Source: CAD feature listing. Evaluate the final solid. Frame: model axes, mm. A direction names the side the tool comes from. Round coordinates to 2 decimals unless told otherwise and drop trailing zeros. Order: outer loops, then holes, each group sorted by start corner. A loop starts at its lowest first (then second) coordinate and runs counter-clockwise, first axis right, second up. Notation, with made-up numbers: M 78,-26.75 L 114,-26.75 A13 cw 114,-14.75 Z; hole C 66.25,74.5 d6. An arc over 180 degrees is marked long. Use CSV: the item, a comma, the result in double quotes. Start each with the question number.
```python
from build123d import *

# Parameters (mm, degrees)
SKETCH1_W           = 24
SKETCH1_H           = 24
SKETCH1_R           = 2.1
BOSS_EXTRUDE1_DEPTH = 2
SKETCH2_W           = 24
SKETCH2_H           = 26
SKETCH2_R           = 2
BOSS_EXTRUDE2_DEPTH = 2


with BuildPart() as part:
    # Sketch1 → Boss-Extrude1 (new body)
    with BuildSketch(Plane(origin=(0, 0, 0), x_dir=(1, 0, 0), z_dir=(0, 1, 0))):
        with Locations((12, 0)):
            Rectangle(SKETCH1_W, SKETCH1_H)
        with Locations(Location((4, 8, 0), (0, 0, 270))):
            Circle(SKETCH1_R, mode=Mode.SUBTRACT)
        with Locations(Location((12, 8, 0), (0, 0, 270))):
            Circle(SKETCH1_R, mode=Mode.SUBTRACT)
        with Locations(Location((20, 8, 0), (0, 0, 270))):
            Circle(SKETCH1_R, mode=Mode.SUBTRACT)
        with Locations(Location((12, 0, 0), (0, 0, 270))):
            Circle(SKETCH1_R, mode=Mode.SUBTRACT)
        with Locations(Location((20, 0, 0), (0, 0, 270))):
            Circle(SKETCH1_R, mode=Mode.SUBTRACT)
        with Locations(Location((12, -8, 0), (0, 0, 270))):
            Circle(SKETCH1_R, mode=Mode.SUBTRACT)
        with Locations(Location((20, -8, 0), (0, 0, 270))):
            Circle(SKETCH1_R, mode=Mode.SUBTRACT)
        with Locations(Location((4, 0, 0), (0, 0, 270))):
            Circle(SKETCH1_R, mode=Mode.SUBTRACT)
        with Locations(Location((4, -8, 0), (0, 0, 270))):
            Circle(SKETCH1_R, mode=Mode.SUBTRACT)
    extrude(amount=BOSS_EXTRUDE1_DEPTH)

    # Sketch2 → Boss-Extrude2 (add)
    with BuildSketch(Plane.ZY):
        with Locations((0, 13)):
            Rectangle(SKETCH2_W, SKETCH2_H)
        with Locations((-8, 21.666666667)):
            Circle(SKETCH2_R, mode=Mode.SUBTRACT)
        with Locations((0, 21.666666667)):
            Circle(SKETCH2_R, mode=Mode.SUBTRACT)
        with Locations((8, 21.666666667)):
            Circle(SKETCH2_R, mode=Mode.SUBTRACT)
        with Locations((0, 13.666666667)):
            Circle(SKETCH2_R, mode=Mode.SUBTRACT)
        with Locations((8, 13.666666667)):
            Circle(SKETCH2_R, mode=Mode.SUBTRACT)
        with Locations((0, 5.666666667)):
            Circle(SKETCH2_R, mode=Mode.SUBTRACT)
        with Locations((8, 5.666666667)):
            Circle(SKETCH2_R, mode=Mode.SUBTRACT)
        with Locations((-8, 13.666666667)):
            Circle(SKETCH2_R, mode=Mode.SUBTRACT)
        with Locations((-8, 5.666666667)):
            Circle(SKETCH2_R, mode=Mode.SUBTRACT)
    extrude(amount=BOSS_EXTRUDE2_DEPTH)


solid = part.part
```
(1) Reachability of faces 4 (the face through (9, 2, 0)), 5 (the face through (-0.99, 13.75, 6)) from +Z, -Z, +X, -X, +Y, -Y: full face, straight path, thin tool, end or side. Return the list, or none.
(2) Section A-A on x = 20. Return loops of the section in (y, z), plus the area to 3 significant figures.
(3) Contact query for flat-ended pins moving along their axis: P1, Ø4.5, axis at y = 5.67, z = 8, coming from the +X side; P2, Ø12, axis at x = 13, z = -1.5, coming from the +Y side. Output: stop coordinate, or through.
(4) Draft query along Y for faces 1 (the face through (5, 1, 12)), 2 (the face through (11.2, 0, 2.5)), 3 (the face through (-0.986, 4.45, -9.587)). Return one class per face: pulls with the +Y half, pulls with the -Y half, needs draft (parallel to the pull), parting line crosses it, or undercut.
(5) Line query: line 1 along Y through (x, z) = (-0.45, -8); line 2 along X through (y, z) = (0.65, 8); line 3 along X through (y, z) = (6.5, 2). Output: solid intervals per line, ascending.
(6) Section C-C on y = 15. Return loops of the section in (x, z).
(7) Section B-B on z = 0. Give the number of separate pieces and of enclosed holes in the cut face, plus the area to 3 significant figures.
Results below:
1,face 4,"+Z, -Z, +X, +Y"
1,face 5,"+X, -X"
2,outline,"M 0,-12 L 2,-12 L 2,-10.1 L 0,-10.1 Z; M 0,-5.9 L 2,-5.9 L 2,-2.1 L 0,-2.1 Z; M 0,2.1 L 2,2.1 L 2,5.9 L 0,5.9 Z; M 0,10.1 L 2,10.1 L 2,12 L 0,12 Z"
2,area,"22.8 mm2"
3,P1,"stops at x = 0"
3,P2,"stops at y = 2"
4,face 1,"needs draft"
4,face 2,"pulls with the -Y half"
4,face 3,"undercut"
5,line 1,"y = 0 to 3.67, 7.67 to 11.67, 15.67 to 19.67, 23.67 to 26"
5,line 2,"x = -2 to 1.9, 6.1 to 9.9, 14.1 to 17.9, 22.1 to 24"
5,line 3,"x = -2 to 0"
6,outline,"M -2,-12 L 0,-12 L 0,-9.49 L -2,-9.49 Z; M -2,-6.51 L 0,-6.51 L 0,-1.49 L -2,-1.49 Z; M -2,1.49 L 0,1.49 L 0,6.51 L -2,6.51 Z; M -2,9.49 L 0,9.49 L 0,12 L -2,12 Z"
7,separate pieces,"7"
7,enclosed holes,"0"
7,area,"50.8 mm2"
